Print and shaded views of the part. All mm, measured from the part's lowest x, y and z. Coordinates: 2 decimals unless noted, no trailing zeros. Write each loop counter-clockwise with the first axis right and the second up, starting at its lowest first coordinate (ties: lowest second). Pieces come first, ordered by that corner, then holes. Notation, with made-up numbers: (53, -14) -> (102, -14) arc R20 ccw to (102, 19) -> close; hole circle Ø3 at (-30.75, 8.25). An arc over 180 degrees is marked (long way). Write item = value, one per line.
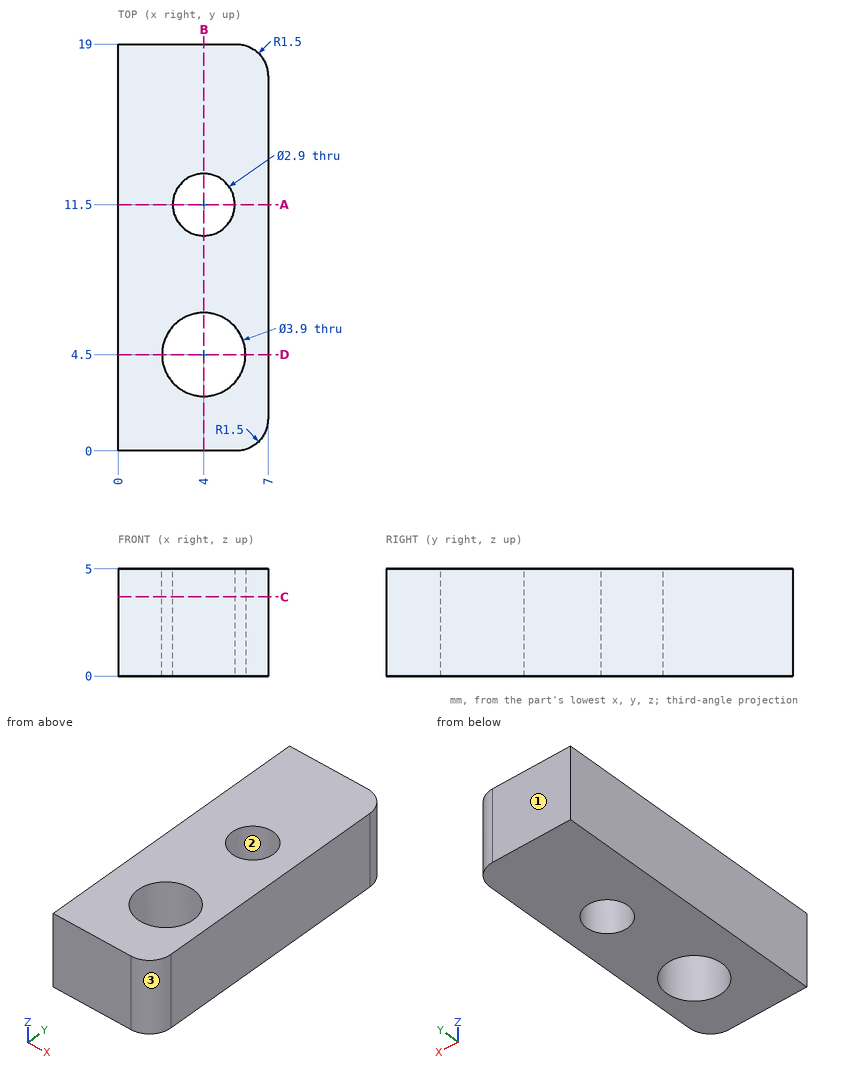
Q1. Saw through at C-C on z = 3.7. Give the cut face in (x, y), and give its area (3 significant figures).
Model answer:
outline = (0, 0) -> (5.5, 0) arc R1.5 ccw to (7, 1.5) -> (7, 17.5) arc R1.5 ccw to (5.5, 19) -> (0, 19) -> close; hole circle Ø3.9 at (4, 4.5); hole circle Ø2.9 at (4, 11.5)
area = 113 mm²
Q2. Saw through at B-B on x = 4. Give the cut face in (y, z), and give its area (3 significant figures).
Model answer:
outline = (0, 0) -> (2.55, 0) -> (2.55, 5) -> (0, 5) -> close; (6.45, 0) -> (10.05, 0) -> (10.05, 5) -> (6.45, 5) -> close; (12.95, 0) -> (19, 0) -> (19, 5) -> (12.95, 5) -> close
area = 61.0 mm²
Q3. Probe line 1 (Y direction, x = 4, z = 1.25); line 2 (Y direction, x = 4.75, z = 4.6); line 3 (X direction, y = 4, z = 4.65). List the from-to ranges inside material, lowest first. Write a range as from..to.
Model answer:
line_1 = 0..2.55, 6.45..10.05, 12.95..19
line_2 = 0..2.7, 6.3..10.26, 12.74..19
line_3 = 0..2.12, 5.88..7
Q4. Saw through at D-D on y = 4.5. Give the cut face in (x, z).
Model answer:
outline = (0, 0) -> (2.05, 0) -> (2.05, 5) -> (0, 5) -> close; (5.95, 0) -> (7, 0) -> (7, 5) -> (5.95, 5) -> close
Q5. Pin check, flat tip, straight feed: pin 1 (2.5 mm diameter, centred on x = 4, y = 11.5, fed in from +Z). Stop position of the tip, or through.
Model answer:
pin_1 = through
Q6. Saw through at A-A on y = 11.5. Give the cut face in (x, z).
Model answer:
outline = (0, 0) -> (2.55, 0) -> (2.55, 5) -> (0, 5) -> close; (5.45, 0) -> (7, 0) -> (7, 5) -> (5.45, 5) -> close
Q7. Mould opens along Y. For the marked faces 1, 2 and 3 say: released by +Y, released by -Y, zero draft, split by the parting line, or undercut.
Model answer:
face_1 = released by +Y
face_2 = undercut
face_3 = released by -Y
